from build123d import *

# Parameters (mm, degrees)
F0_R     = 5
F1_DEPTH = 37
F2_R     = 4.3
F3_DEPTH = 2
F4_R     = 2.6
F5_DEPTH = 15
F7_DEPTH = 11


with BuildPart() as f1:
    # F0 (on Top) → F1 (new body)
    with BuildSketch(Plane.XY):
        Circle(F0_R)
    extrude(amount=F1_DEPTH)

    # F2 (on face) → F3 (cut)
    with BuildSketch(Plane(origin=(0, 0, 0), x_dir=(1, 0, 0), z_dir=(0, 0, -1))):
        Circle(F2_R)
    extrude(amount=-F3_DEPTH, mode=Mode.SUBTRACT)

    # F4 (on face) → F5 (cut)
    with BuildSketch(Plane(origin=(0, 0, 2), x_dir=(1, 0, 0), z_dir=(0, 0, -1))):
        Circle(F4_R)
    extrude(amount=-F5_DEPTH, mode=Mode.SUBTRACT)

    # F6 (on face) → F7 (cut)
    with BuildSketch(Plane(origin=(0, 0, 0), x_dir=(1, 0, 0), z_dir=(0, 0, -1))):
        with BuildLine():
            Line((0, 5), (0, 0))
            Line((0, 0), (2.5, -4.330127))
            ThreePointArc((2.5, -4.330127), (4.829629, 1.294095), (0, 5))
        make_face()
    extrude(amount=-F7_DEPTH, mode=Mode.SUBTRACT)


solid = f1.part
Could you check a few things on this model? Use its own coordinates, in mm. A direction names the side the tool comes from. Give positions to 0.01 mm unless a question says otherwise; leave off trailing zeros. Order: outer loops, then holes, each group sorted by start corner. A loop starts at its lowest first (then second) coordinate and runs counter-clockwise, first axis right, second up. Notation, with made-up numbers: (37.25, 56) - (81.25, 56) arc R33 ccw to (81.25, 92) - close; hole circle Ø4 at (14.5, 88.25). An arc over 180 degrees is marked (long way). One line per question, with ' | ' between items. Start each with the question number.
Item 1: Thinking about a two-plate mould opening in Y: for faces 4 (the cylindrical face through (-2.6, -0.1, 9.4)), 5 (the flat face through (-4, 2, 0)), 6 (the flat face through (1.892, 3.276, 6.645)), which applies, pulls with the +Y half, pulls with the -Y half, needs draft (parallel to the pull), parting line crosses it, or undercut?
Item 2: I want a section at D-D on z = 5.5. Write out the boundary of the cut face in (x, y).
Item 3: I want a section at B-B on x = -1.25. Write out the boundary of the cut face in (y, z).
Item 4: I need wall thicknesses on probe 1 along X at (y, z) = (0, 12); probe 2 along X at (y, z) = (0, 6.5). Which ranges of each line are inside material? Lowest first, please. Write a range as [from, to].
Item 5: I want a section at A-A on y = 0. Write out the boundary of the cut face in (x, z), then the cut area to 3 significant figures.
Item 6: I want a section at C-C on z = 15.5. Write out the boundary of the cut face in (x, y).
Item 7: I'm going to push flat-ended pins straight in: pin 1 Ø5.5 at (x, y) = (0.5, -1) entering from -Z; pin 2 Ø1.5 at (y, z) = (3, 7.5) entering from +X; pin 3 Ø2 at (x, z) = (-2, 24.5) entering from +Y. Where does each tip first touch, or does it pass through?
Item 8: For faces 1 (the flat face through (-3, 1, 2)), 2 (the flat face through (0, 0, 37)), 3 (the flat face through (3, 0, 11)), which set-ups out of +Z, -Z, +X, -X, +Y, -Y let a thin tool reach every point of the face, with its end or its side?
Verdict:
1) face 4: undercut | face 5: needs draft | face 6: pulls with the -Y half
2) outline: (0, -5) - (0, -2.6) arc R2.6 cw (long way) to (1.3, 2.25) - (2.5, 4.33) arc R5 ccw (long way) to start
3) outline: (-4.84, 0) - (-4.11, 0) - (-4.11, 2) - (-2.28, 2) - (-2.28, 17) - (2.28, 17) - (2.28, 2) - (4.11, 2) - (4.11, 0) - (4.84, 0) - (4.84, 37) - (-4.84, 37) - close
4) probe 1: [-5, -2.6], [2.6, 5] | probe 2: [-5, -2.6]
5) outline: (-5, 0) - (-4.3, 0) - (-4.3, 2) - (-2.6, 2) - (-2.6, 17) - (2.6, 17) - (2.6, 11) - (5, 11) - (5, 37) - (-5, 37) - close | area: 252 mm^2
6) outline: circle Ø10 at (0, 0); hole circle Ø5.2 at (0, 0)
7) pin 1: z = 2 | pin 2: x = 2.17 | pin 3: y = 4.9
8) face 1: -Z | face 2: +Z, +X, -X, +Y, -Y | face 3: -Z, +X, -Y
